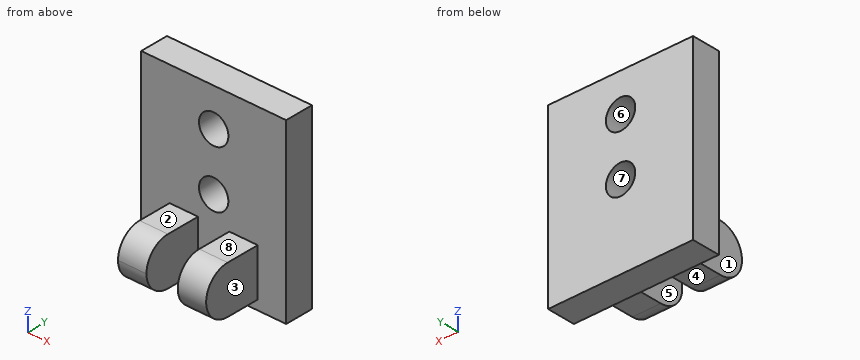
```python
from build123d import *

# Parameters (mm, degrees)
F0_W     = 15.3
F0_H     = 18.7374445884
F1_DEPTH = 3
F2_W     = 3
F2_H     = 5
F3_DEPTH = 3.5
F5_R     = 1.55
F6_DEPTH = 5
F7_DEPTH = 3
F9_DEPTH = 3


with BuildPart() as f1:
    # F0 (on Front) → F1 (new body)
    with BuildSketch(Plane.XZ):
        Rectangle(F0_W, F0_H)
    extrude(amount=F1_DEPTH)

    # F2 (on face) → F3 (join)
    with BuildSketch(Plane.XZ.offset(3)):
        with Locations((-3.15, -5.8687222942)):
            Rectangle(F2_W, F2_H)
        with Locations((3.15, -5.8687222942)):
            Rectangle(F2_W, F2_H)
    extrude(amount=F3_DEPTH)

    # F5 (on face) → F6 (cut)
    with BuildSketch(Plane.XZ.offset(3)):
        with Locations((0, -0.6312777058)):
            Circle(F5_R)
        with Locations((0, 5.3687222942)):
            Circle(F5_R)
    extrude(amount=-F6_DEPTH, mode=Mode.SUBTRACT)

    # F4 (on face) → F7 (join)
    with BuildSketch(Plane(origin=(-4.65, 0, 0), x_dir=(0, -1, 0), z_dir=(-1, 0, 0))):
        with BuildLine():
            ThreePointArc((6.5, -8.3687222942), (8.267766953, -7.6364892472), (9, -5.8687222942))
            ThreePointArc((9, -5.8687222942), (8.267766953, -4.1009553413), (6.5, -3.3687222942))
            Line((6.5, -3.3687222942), (6.5, -8.3687222942))
        make_face()
    extrude(amount=-F7_DEPTH)

    # F8 (on face) → F9 (join)
    with BuildSketch(Plane.YZ.offset(4.65)):
        with BuildLine():
            ThreePointArc((-6.5, -8.3687222942), (-4.732233047, -7.6364892472), (-4, -5.8687222942))
            ThreePointArc((-4, -5.8687222942), (-4.732233047, -4.1009553413), (-6.5, -3.3687222942))
            Line((-6.5, -3.3687222942), (-6.5, -8.3687222942))
        make_face()
        with BuildLine():
            Line((-6.5, -8.3687222942), (-6.5, -3.3687222942))
            ThreePointArc((-6.5, -3.3687222942), (-9, -5.8687222942), (-6.5, -8.3687222942))
        make_face()
    extrude(amount=-F9_DEPTH)


solid = f1.part
```
For this review, take the finished solid that the model builds, in its own axes (mm). Face numbers are marked on the shaded views. A direction names the side the tool comes from. Round coordinates to 2 decimals unless told otherwise and drop trailing zeros. Order: outer loops, then holes, each group sorted by start corner. A loop starts at its lowest first (then second) coordinate and runs counter-clockwise, first axis right, second up.
Q1. We need section D-D, the plane z = 5. Give the boundary of the cut face in (x, y).
Findings below:
outline: (-7.65, -3) - (-1.51, -3) - (-1.51, 0) - (-7.65, 0) - close; (1.51, -3) - (7.65, -3) - (7.65, 0) - (1.51, 0) - close
Q2. We need section C-C, the plane x = -2. Give the boundary of the cut face in (y, z).
Findings below:
outline: (-6.5, -8.37) - (-3, -8.37) - (-3, -9.37) - (0, -9.37) - (0, 9.37) - (-3, 9.37) - (-3, -3.37) - (-6.5, -3.37) arc R2.5 ccw to start
Q3. We need section B-B, the plane y = -3.25. Give the boundary of the cut face in (x, z), plus the area to 3 significant figures.
Findings below:
outline: (-4.65, -8.37) - (-1.65, -8.37) - (-1.65, -3.37) - (-4.65, -3.37) - close; (1.65, -8.37) - (4.65, -8.37) - (4.65, -3.37) - (1.65, -3.37) - close
area: 30.0 mm2
Q4. Insertion check: P1, Ø1.5, axis at x = 3, y = -5.5, coming from the -Z side; P2, Ø4, axis at y = -6, z = -6, coming from the +X side; P3, Ø5, axis at x = 4.5, z = 5, coming from the -Y side. Each pin has a flat end and moves straight along its axis. Give the tip position at first contact, or say it passes through.
Findings below:
P1: stops at z = -8.37
P2: stops at x = 4.65
P3: stops at y = -3
Q5. Mouldability with a two-part tool opening along Z and no side actions: class the marked faces 5, 6, 7 and 8 as pulls with the +Z half, pulls with the -Z half, needs draft (parallel to the pull), parting line crosses it, or undercut.
Findings below:
face 5: needs draft
face 6: undercut
face 7: undercut
face 8: pulls with the +Z half
Q6. We need section A-A, the plane x = 0. Give the boundary of the cut face in (y, z).
Findings below:
outline: (-3, -9.37) - (0, -9.37) - (0, -2.18) - (-3, -2.18) - close; (-3, 0.92) - (0, 0.92) - (0, 3.82) - (-3, 3.82) - close; (-3, 6.92) - (0, 6.92) - (0, 9.37) - (-3, 9.37) - close
Q7. Wall thickness on line 1 (Z direction, x = 0, y = -0.7); line 2 (X direction, y = -7.5, z = -7.75); line 3 (Y direction, x = 4.75, z = -3.75): over which ranges is each line inside the solid? List them lowest first.
Findings below:
line 1: z = -9.37 to -2.18, 0.92 to 3.82, 6.92 to 9.37
line 2: x = -4.65 to -1.65, 1.65 to 4.65
line 3: y = -3 to 0
Q8. Machinability: for the marked faces 1, 2, 3 and 4, which of the approach directions +Z, -Z, +X, -X, +Y, -Y give a long, thin tool a straight path to every point of the face, cutting with its end or side? Answer none if there is none.
Findings below:
face 1: +Z, -Z, -X, -Y
face 2: +Z, +X, -X, -Y
face 3: +Z, -Z, +X, -Y
face 4: -Z, +X, -X, -Y
